Work out the finished part from the listing and answer in its coordinate system (mm). A direction names the side the tool comes from. Give positions to 0.01 mm unless a question says otherwise; leave off trailing zeros. Order: outer loops, then holes, each group sorted by start corner. A loop starts at its lowest first (then second) coordinate and runs counter-clockwise, first axis right, second up. Notation, with made-up numbers: (50, 11) - (79, 11) arc R26 ccw to (79, 26) - close; hole circle Ø9 at (-8, 78). An arc over 180 degrees is marked (long way). Put each result on its own line as item: value.
```python
from build123d import *

# Parameters (mm, degrees)
ESBO_O1_W                = 40
ESBO_O1_H                = 62
RESSALTO_EXTRUS_O1_DEPTH = 6
ESBO_O2_W                = 21
ESBO_O2_H                = 10
RESSALTO_EXTRUS_O2_DEPTH = 48
CHANFRO1_SIZE            = 6
ESBO_O3_W                = 10
ESBO_O3_H                = 62
RESSALTO_EXTRUS_O3_DEPTH = 20
ESBO_O4_W                = 62
ESBO_O4_H                = 10
RESSALTO_EXTRUS_O4_DEPTH = 50
ESBO_O5_W                = 2
ESBO_O5_H                = 13
RESSALTO_EXTRUS_O5_DEPTH = 10
ESBO_O6_W                = 20
ESBO_O6_H                = 3
ESBO_O6_H_2              = 2.5
CORTE_EXTRUS_O1_DEPTH    = 92.433035605
CHANFRO2_SIZE            = 1
CHANFRO3_SIZE            = 5
ESBO_O7_W                = 62
ESBO_O7_H                = 26
RESSALTO_EXTRUS_O6_DEPTH = 10
CHANFRO4_SIZE            = 0.5
ESBO_O8_W                = 62
ESBO_O8_H                = 6
RESSALTO_EXTRUS_O7_DEPTH = 20


with BuildPart() as part:
    # Esboço1 → Ressalto-extrusão1 (new body)
    with BuildSketch(Plane(origin=(0, 0, 0), x_dir=(1, 0, 0), z_dir=(0, 1, 0))):
        Rectangle(ESBO_O1_W, ESBO_O1_H)
    extrude(amount=RESSALTO_EXTRUS_O1_DEPTH)

    # Esboço2 → Ressalto-extrusão2 (add)
    with BuildSketch(Plane(origin=(0, 6, 0), x_dir=(1, 0, 0), z_dir=(0, 1, 0))):
        with Locations((0, -26)):
            Rectangle(ESBO_O2_W, ESBO_O2_H)
        with Locations((0, 26)):
            Rectangle(ESBO_O2_W, ESBO_O2_H)
    extrude(amount=RESSALTO_EXTRUS_O2_DEPTH)

    # Chanfro1
    chanfro1_edges = [part.edges().sort_by_distance(p)[0] for p in [
        (0, 6, -21),
        (0, 6, 21),
    ]]
    chamfer(chanfro1_edges, length=CHANFRO1_SIZE)

    # Esboço3 → Ressalto-extrusão3 (add)
    with BuildSketch(Plane.XZ):
        with Locations((-15, 0)):
            Rectangle(ESBO_O3_W, ESBO_O3_H)
    extrude(amount=RESSALTO_EXTRUS_O3_DEPTH)

    # Esboço4 → Ressalto-extrusão4 (add)
    with BuildSketch(Plane(origin=(-10, 0, 0), x_dir=(0, 0, -1), z_dir=(1, 0, 0))):
        with Locations((0, -15)):
            Rectangle(ESBO_O4_W, ESBO_O4_H)
    extrude(amount=RESSALTO_EXTRUS_O4_DEPTH)

    # Esboço5 → Ressalto-extrusão5 (add)
    with BuildSketch(Plane.XY.offset(31)):
        with Locations((-11.5, 47.5)):
            Rectangle(ESBO_O5_W, ESBO_O5_H)
        with Locations((11.5, 47.5)):
            Rectangle(ESBO_O5_W, ESBO_O5_H)
    ressalto_extrus_o5 = extrude(amount=-RESSALTO_EXTRUS_O5_DEPTH)

    # Espelhar1: Ressalto-extrusão5 across plane
    add(ressalto_extrus_o5.mirror(Plane.XY))

    # Esboço6 → Corte-extrusão1 (cut, through all)
    with BuildSketch(Plane.XY.offset(31)):
        with Locations((0, 47.5)):
            Rectangle(ESBO_O6_W, ESBO_O6_H)
        with Locations((0, 1.25)):
            Rectangle(ESBO_O6_W, ESBO_O6_H_2)
    extrude(amount=-CORTE_EXTRUS_O1_DEPTH, mode=Mode.SUBTRACT)

    # Chanfro2
    chanfro2_edges = [part.edges().sort_by_distance(p)[0] for p in [
        (0, 46, -31),
        (0, 46, 31),
        (0, 2.5, -31),
        (0, 2.5, 31),
    ]]
    chamfer(chanfro2_edges, length=CHANFRO2_SIZE)

    # Chanfro3
    # the kernel refuses this chamfer: 5 mm, written as the material it adds along each edge
    with BuildSketch(Plane(origin=(-10.5, 41, -31), x_dir=(-0.9996219169112968, 0.027495876610586317, 0), z_dir=(0, 0, 1))) as chanfro3_piece_1_section:
        Polygon((CHANFRO3_SIZE * 0.999621916911, CHANFRO3_SIZE * 0.0274958766106), (-CHANFRO3_SIZE * 0.0274958766106, CHANFRO3_SIZE * 0.999621916911), (0, 0), align=None)
    chanfro3_piece_1 = extrude(amount=10, mode=Mode.PRIVATE)
    chanfro3_piece_1 = split(chanfro3_piece_1, bisect_by=Plane(origin=(-12.5, 38.93054755, -26), z_dir=(1, 0, 0)), keep=Keep.TOP, mode=Mode.PRIVATE)
    add(chanfro3_piece_1)
    with BuildSketch(Plane(origin=(10.5, 41, -31), x_dir=(-0.02749587661058701, -0.9996219169112968, 0), z_dir=(0, 0, 1))) as chanfro3_piece_2_section:
        Polygon((CHANFRO3_SIZE * 0.999621916911, CHANFRO3_SIZE * 0.0274958766106), (-CHANFRO3_SIZE * 0.0274958766106, CHANFRO3_SIZE * 0.999621916911), (0, 0), align=None)
    chanfro3_piece_2 = extrude(amount=10, mode=Mode.PRIVATE)
    chanfro3_piece_2 = split(chanfro3_piece_2, bisect_by=Plane(origin=(12.5, 38.93054755, -26), z_dir=(-1, 0, 0)), keep=Keep.TOP, mode=Mode.PRIVATE)
    add(chanfro3_piece_2)
    with BuildSketch(Plane(origin=(10.5, 41, 31), x_dir=(0.9996219169112968, 0.027495876610586317, 0), z_dir=(0, 0, -1))) as chanfro3_piece_3_section:
        Polygon((CHANFRO3_SIZE * 0.999621916911, CHANFRO3_SIZE * 0.0274958766106), (-CHANFRO3_SIZE * 0.0274958766106, CHANFRO3_SIZE * 0.999621916911), (0, 0), align=None)
    chanfro3_piece_3 = extrude(amount=10, mode=Mode.PRIVATE)
    chanfro3_piece_3 = split(chanfro3_piece_3, bisect_by=Plane(origin=(12.5, 38.93054755, 26), z_dir=(-1, 0, 0)), keep=Keep.TOP, mode=Mode.PRIVATE)
    add(chanfro3_piece_3)
    with BuildSketch(Plane(origin=(-10.5, 41, 31), x_dir=(0.027495876610584936, -0.9996219169112968, 0), z_dir=(0, 0, -1))) as chanfro3_piece_4_section:
        Polygon((CHANFRO3_SIZE * 0.999621916911, CHANFRO3_SIZE * 0.0274958766106), (-CHANFRO3_SIZE * 0.0274958766106, CHANFRO3_SIZE * 0.999621916911), (0, 0), align=None)
    chanfro3_piece_4 = extrude(amount=10, mode=Mode.PRIVATE)
    chanfro3_piece_4 = split(chanfro3_piece_4, bisect_by=Plane(origin=(-12.5, 38.93054755, 26), z_dir=(1, 0, 0)), keep=Keep.TOP, mode=Mode.PRIVATE)
    add(chanfro3_piece_4)

    # Esboço7 → Ressalto-extrusão6 (add)
    with BuildSketch(Plane.ZY.offset(20)):
        with Locations((0, -7)):
            Rectangle(ESBO_O7_W, ESBO_O7_H)
    extrude(amount=RESSALTO_EXTRUS_O6_DEPTH)

    # Chanfro4
    chanfro4_edges = [part.edges().sort_by_distance(p)[0] for p in [
        (-10.5, 6, -23),
        (10.5, 6, -23),
        (10.5, 6, 23),
        (-10.5, 6, 23),
    ]]
    chamfer(chanfro4_edges, length=CHANFRO4_SIZE)

    # Esboço8 → Ressalto-extrusão7 (add)
    with BuildSketch(Plane(origin=(20, 0, 0), x_dir=(0, 0, -1), z_dir=(1, 0, 0))):
        with Locations((0, 3)):
            Rectangle(ESBO_O8_W, ESBO_O8_H)
    extrude(amount=RESSALTO_EXTRUS_O7_DEPTH)


solid = part.part
```
(1) Section B-B, the plane x = 15.5 is taken. Write down the section's boundary in (y, z), then the cut area to 3 significant figures.
Geometry check:
outline: (-20, -31) - (-10, -31) - (-10, 31) - (-20, 31) - close; (0, -31) - (6, -31) - (6, 31) - (0, 31) - close
area: 992 mm²
(2) Given pin 1 (17 mm diameter, centred on y = 27, z = -20.5, fed in from +X); pin 2 (17 mm diameter, centred on y = 15.5, z = -26, fed in from -X); pin 3 (4.5 mm diameter, centred on y = 47, z = 28, fed in from +X), each flat-ended and moving along its own axis, determine where each tip first touches the part or whether it passes through.
Geometry check:
pin 1: stops at x = 10.5
pin 2: stops at x = -10.5
pin 3: stops at x = 12.5
(3) Determine the mould class of faces 1 (the face through (0, 9, 18)), 2 (the face through (-11.5, 37, 26.1)), 3 (the face through (11.5, 37, -26.1)), 4 (the face through (-10, 47, 26)) for opening direction X: pulls with the +X half, pulls with the -X half, needs draft (parallel to the pull), parting line crosses it, or undercut.
Geometry check:
face 1: needs draft
face 2: pulls with the -X half
face 3: pulls with the +X half
face 4: undercut
(4) Section A-A, the plane y = 10 is taken. Write down the section's boundary in (x, z), then the cut area to 3 significant figures.
Geometry check:
outline: (-10.5, -31) - (10.5, -31) - (10.5, -19) - (-10.5, -19) - close; (-10.5, 19) - (10.5, 19) - (10.5, 31) - (-10.5, 31) - close
area: 504 mm²
(5) Section D-D, the plane x = -6.5 is taken. Write down the section's boundary in (y, z).
Geometry check:
outline: (-20, -31) - (-10, -31) - (-10, 31) - (-20, 31) - close; (2.5, -30) - (3.5, -31) - (45, -31) - (46, -30) - (46, -21) - (12, -21) - (6, -15) - (6, 15) - (12, 21) - (46, 21) - (46, 30) - (45, 31) - (3.5, 31) - (2.5, 30) - close; (49, -31) - (54, -31) - (54, -21) - (49, -21) - close; (49, 21) - (54, 21) - (54, 31) - (49, 31) - close
(6) A tool of negligible diameter and unlimited length cuts with its end or side. For faces 5 (the face through (0, 46, 26)), 6 (the face through (0, 33, 21)), 7 (the face through (10.5, 21, -25)), from which of +Z, -Z, +X, -X, +Y, -Y can it reach the whole face along a straight path? Write none if from no direction.
Geometry check:
face 5: +Z, -Z
face 6: +X, -X, +Y
face 7: +Z, -Z, +X
(7) Straight lines are drawn through the part: line 1 (Y direction, x = -7, z = 0.5); line 2 (Z direction, x = -10.5, y = 41); line 3 (Y direction, x = 18.5, z = -6.5). For each, find the intervals that lie inside material, in ascending order.
Geometry check:
line 1: y = -20 to -10, 2.5 to 6
line 2: z = -31 to -21, 21 to 31
line 3: y = -20 to -10, 0 to 6
(8) Section C-C, the plane z = -20 is taken. Write down the section's boundary in (x, y), then the cut area to 3 significant figures.
Geometry check:
outline: (-30, -20) - (40, -20) - (40, -10) - (-10, -10) - (-10, 2.5) - (10, 2.5) - (10, 0) - (40, 0) - (40, 6) - (11, 6) - (10.5, 6.5) - (10.5, 11) - (-10.5, 11) - (-10.5, 6.5) - (-11, 6) - (-30, 6) - close
area: 1,380 mm²
